Read the model definition and answer for the solid it produces. Units are mm, in the model's axes. A direction names the side the tool comes from. Round coordinates to 2 decimals unless told otherwise and drop trailing zeros. Write each loop counter-clockwise with the first axis right and the second up, starting at its lowest first coordinate (ties: lowest second). Pieces come first, ordered by that corner, then holes. Notation, with made-up numbers: (-36, 25.5) -> (15, 25.5) arc R24 cw to (15, 35.5) -> close; hole circle Ø3 at (82, 9). An arc over 180 degrees is marked (long way). Return JSON: item names as keys, results as strings. Group by question number.
(1) Given pin 1 (1.3 mm diameter, centred on x = 1.5, y = 11.5, fed in from +Z); pin 2 (12 mm diameter, centred on y = 14, z = 33.5, fed in from -X); pin 3 (6 mm diameter, centred on x = -4, y = 18, fed in from +Z); pin 4 (2.5 mm diameter, centred on x = 17, y = 15, fed in from +Z), each flat-ended and moving along its own axis, determine where each tip first touches the part or whether it passes through.
(2) A cutting plane is placed at D-D on z = 46. Give the vertices of the cut face in (x, y), then the cut area to 3 significant figures.
(3) A cutting plane is placed at C-C on x = 25.5. Give the vertices of the cut face in (y, z), then the cut area to 3 significant figures.
(4) Straight lines are drawn through the part: line 1 (X direction, y = 6.5, z = 33); line 2 (Z direction, x = 0.5, y = 16.5); line 3 (Z direction, x = 3, y = 19). For each, find the intervals that lie inside material, in ascending order.
(5) For faces 1 (the cylindrical face through (0.625, 11.082, 48.832)), 2 (the cylindrical face through (-4.4, 8.8, 10.7)), 3 (the flat face through (18.5, 11.4, 37)), determine the directions among +Z, -Z, +X, -X, +Y, -Y from which every point of the face is accessible in a straight line to the end or side of a thin tool.
(6) A cutting plane is placed at A-A on y = 11.25. Give the vertices of the cut face in (x, z).
(7) A cutting plane is placed at B-B on z = 11.2. Give the vertices of the cut face in (x, y), then the cut area to 3 significant figures.
```python
from build123d import *

# Parameters (mm, degrees)
SKETCH_1_W           = 18.8
SKETCH_1_H           = 22.5
EXTRUDE_1_DEPTH      = 37
FILLET_1_R           = 3
SKETCH_2_W           = 5
SKETCH_2_H           = 22.5
EXTRUDE_2_DEPTH      = 27
FILLET_2_R           = 3
EXTRUDE_3_DEPTH      = 9
EXTRUDE_3_DEPTH_BACK = 27.8
SKETCH_3_R           = 2.5


with BuildPart() as part:
    # 草图1 → 凸台-拉伸1 (new body)
    with BuildSketch(Plane.XY):
        with Locations((9.4, 11.25)):
            Rectangle(SKETCH_1_W, SKETCH_1_H)
    extrude(amount=EXTRUDE_1_DEPTH)

    # 圆角1
    fillet_1_edges = [part.edges().sort_by_distance(p)[0] for p in [
        (9.4, 0, 0),
        (9.4, 22.5, 0),
    ]]
    fillet(fillet_1_edges, radius=FILLET_1_R)

    # 草图2 → 凸台-拉伸2 (add)
    with BuildSketch(Plane.XY.offset(37)):
        with Locations((6.75562561, 11.25)):
            Rectangle(SKETCH_2_W, SKETCH_2_H)
        with Locations((11.75562561, 11.25)):
            Rectangle(SKETCH_2_W, SKETCH_2_H)
        with BuildLine():
            Line((14.25562561, 22.5), (14.25562561, 0))
            ThreePointArc((14.25562561, 0), (17.943444104, 11.25), (14.25562561, 22.5))
        make_face()
        with BuildLine():
            Line((4.25562561, 22.5), (4.25562561, 0))
            ThreePointArc((4.25562561, 0), (0.624004306, 11.25), (4.25562561, 22.5))
        make_face()
    extrude(amount=EXTRUDE_2_DEPTH)

    # 圆角2
    fillet_2_edges = [part.edges().sort_by_distance(p)[0] for p in [
        (9.25562561, 0, 64),
        (17.943444104, 11.25, 64),
        (9.25562561, 22.5, 64),
        (0.624004306, 11.25, 64),
    ]]
    fillet(fillet_2_edges, radius=FILLET_2_R)

    # 草图3 → 凸台-拉伸3 (add, two sides: drawn at the far end of the back side and taken through both)
    with BuildSketch(Plane.ZY.offset(-EXTRUDE_3_DEPTH_BACK)):
        with Locations((11.2, 11.25)):
            Circle(SKETCH_3_R)
    extrude(amount=EXTRUDE_3_DEPTH + EXTRUDE_3_DEPTH_BACK)


solid = part.part
```
Checks:
{
 "1": {"pin 1": "stops at z = 63.61", "pin 2": "stops at x = 0", "pin 3": "passes through", "pin 4": "stops at z = 63.75"},
 "2": {"outline": "(4.26, 0) -> (14.26, 0) arc R19 ccw to (14.26, 22.5) -> (4.26, 22.5) arc R19.24 ccw to start", "area": "337 mm^2"},
 "3": {"outline": "circle Ø5 at (11.25, 11.2)", "area": "19.6 mm^2"},
 "4": {"line 1": "x = 0 to 18.8", "line 2": "z = 0 to 37", "line 3": "z = 0 to 62.9"},
 "5": {"face 1": "+Z, -X", "face 2": "-X", "face 3": "+Z, +X"},
 "6": {"outline": "(-9, 8.7) -> (0, 8.7) -> (0, 0) -> (18.8, 0) -> (18.8, 8.7) -> (27.8, 8.7) -> (27.8, 13.7) -> (18.8, 13.7) -> (18.8, 37) -> (17.94, 37) -> (17.94, 61) arc R3 ccw to (14.94, 64) -> (3.62, 64) arc R3 ccw to (0.62, 61) -> (0.62, 37) -> (0, 37) -> (0, 13.7) -> (-9, 13.7) -> close"},
 "7": {"outline": "(-9, 8.75) -> (0, 8.75) -> (0, 0) -> (18.8, 0) -> (18.8, 8.75) -> (27.8, 8.75) -> (27.8, 13.75) -> (18.8, 13.75) -> (18.8, 22.5) -> (0, 22.5) -> (0, 13.75) -> (-9, 13.75) -> close", "area": "513 mm^2"}
}
